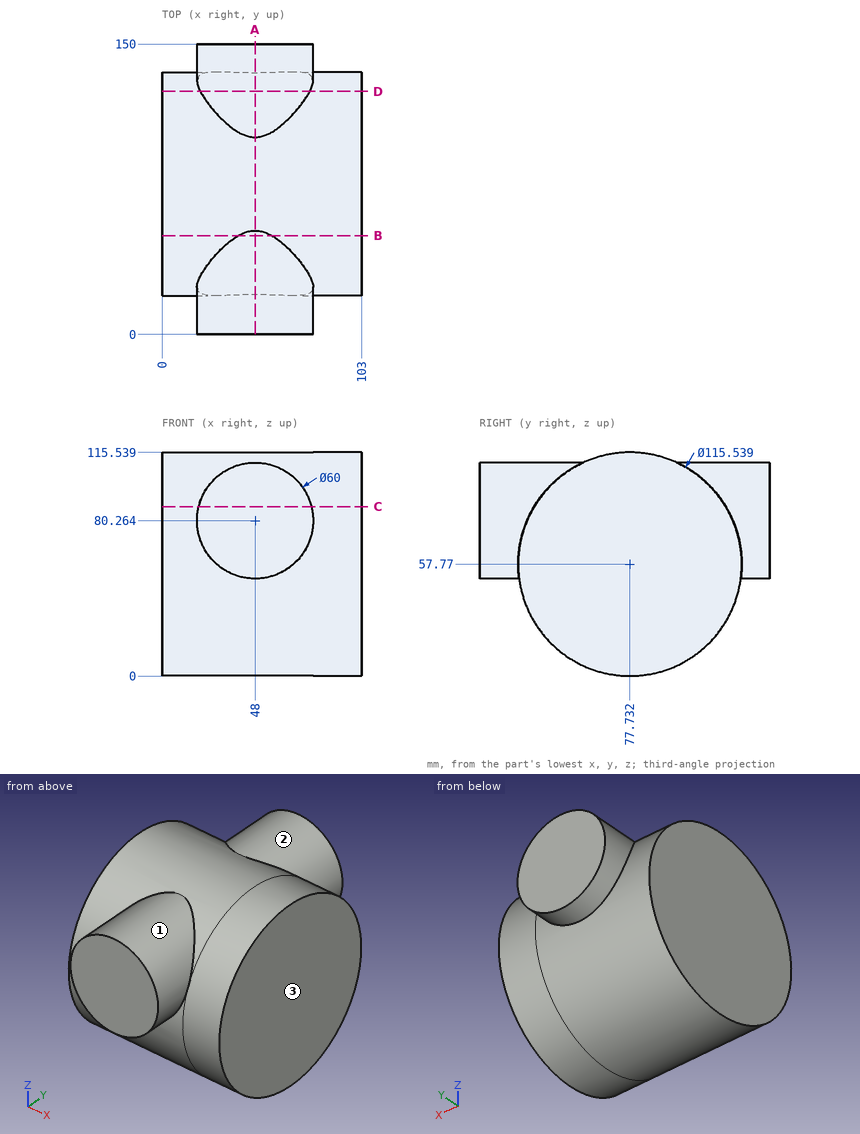
Design review of the part shown in the three views and the two pictorial views. Dimensions are in mm from the part's minimum x, y and z. A direction names the side the tool comes from. Round coordinates to 2 decimals unless told otherwise and drop trailing zeros. Order: outer loops, then holes, each group sorted by start corner. A loop starts at its lowest first (then second) coordinate and runs counter-clockwise, first axis right, second up.
Item 1: For pin 1 (6 mm diameter, centred on x = 86.5, y = 89, fed in from +Z) (1 decimal); pin 2 (6 mm diameter, centred on x = 70.5, y = 74.5, fed in from +Z); pin 3 (2 mm diameter, centred on x = 23, z = 103.5, fed in from -Y) (1 decimal); pin 4 (3 mm diameter, centred on y = 19, z = 61.5, fed in from -X), all flat-tipped, find the tip position at first contact; note any pin that passes through.
Working result:
pin 1: stops at z = 114.9
pin 2: stops at z = 115.54
pin 3: stops at y = 41.2
pin 4: stops at x = 0
Item 2: Machinability: for the marked faces 1, 2 and 3, which of the approach directions +Z, -Z, +X, -X, +Y, -Y give a long, thin tool a straight path to every point of the face, cutting with its end or side? Answer none if there is none.
Working result:
face 1: -Y
face 2: +Y
face 3: +Z, -Z, +X, +Y, -Y
Item 3: To check wall thickness, follow probe 1 along Z at (x, y) = (81, 76) (1 decimal); probe 2 along Z at (x, y) = (45, 69.5); probe 3 along Y at (x, z) = (63, 20) (1 decimal). State the ranges of each line that lie inside material, in increasing order.
Working result:
probe 1: z = 0 to 115.5
probe 2: z = 0.59 to 114.95
probe 3: y = 34 to 121.4
Item 4: Add section D-D, the plane y = 125.5. State the section outline as (x, z) points.
Working result:
outline: (0, 25.28) - (103, 25.28) - (103, 90.26) - (76.29, 90.26) arc R30 ccw to (19.71, 90.26) - (0, 90.26) - close
Item 5: Add section C-C, the plane z = 87.5. State the section outline as (x, y) points (1 decimal).
Working result:
outline: (0, 28.2) - (18.9, 28.2) - (18.9, 0) - (77.1, 0) - (77.1, 28.2) - (103, 28.2) - (103, 127.3) - (77.1, 127.3) - (77.1, 150) - (18.9, 150) - (18.9, 127.3) - (0, 127.3) - close
Item 6: Add section A-A, the plane x = 48. State the section outline as (y, z) points, and give its area (3 significant figures).
Working result:
outline: (0, 50.26) - (20.45, 50.26) arc R57.77 ccw to (135.01, 50.26) - (150, 50.26) - (150, 110.26) - (101.85, 110.26) arc R57.77 ccw to (53.61, 110.26) - (0, 110.26) - close
area: 13,500 mm2
Item 7: Add section B-B, the plane y = 51. State the section outline as (x, z) points.
Working result:
outline: (0, 6.56) - (103, 6.56) - (103, 108.98) - (56.67, 108.98) arc R30 ccw to (39.33, 108.98) - (0, 108.98) - close
